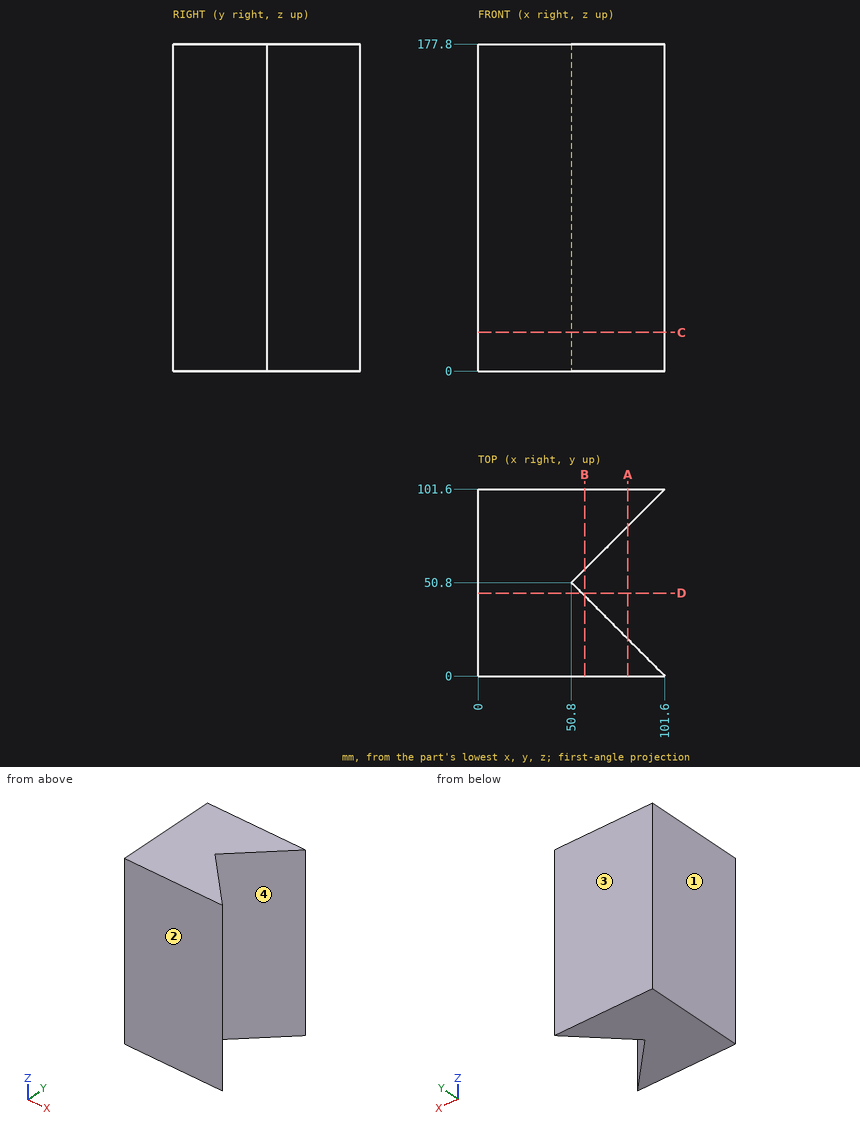
Geometry check sheet. Reference: drawing and pictorial views, mm from the part's lowest x, y, z. Round coordinates to 2 decimals unless told otherwise and drop trailing zeros. Write each loop counter-clockwise with the first axis right and the second up, starting at its lowest first coordinate (ties: lowest second). Pieces come first, ordered by that corner, then holes. Notation, with made-up numbers: (-40, -25.5) -> (-33, -25.5) arc R30 cw to (-33, 6.5) -> close; hole circle Ø10 at (-0.5, 6.5). An arc over 180 degrees is marked (long way). Put each result on its own line as item: value.
1) Cross-section at A-A, the plane x = 81.5. Enter the section's corners in (y, z), plus the area to 3 significant figures.
Recorded:
outline: (0, 0) -> (20.1, 0) -> (20.1, 177.8) -> (0, 177.8) -> close; (81.5, 0) -> (101.6, 0) -> (101.6, 177.8) -> (81.5, 177.8) -> close
area: 7,150 mm2
2) Depth check by flat-ended pin: P1, Ø12, axis at y = 40.5, z = 143.5, coming from the +X side; P2, Ø8, axis at x = 28, y = 47.5, coming from the -Z side. Enter the tip coordinate at first touch or a pass-through.
Recorded:
P1: stops at x = 67.1
P2: stops at z = 0
3) Cross-section at B-B, the plane x = 58. Enter the section's corners in (y, z), plus the area to 3 significant figures.
Recorded:
outline: (0, 0) -> (43.6, 0) -> (43.6, 177.8) -> (0, 177.8) -> close; (58, 0) -> (101.6, 0) -> (101.6, 177.8) -> (58, 177.8) -> close
area: 15,500 mm2
4) Release check for a two-part mould opening along Y. For the marked faces 1, 2, 3 and 4 record: pulls with the +Y half, pulls with the -Y half, needs draft (parallel to the pull), parting line crosses it, or undercut.
Recorded:
face 1: needs draft
face 2: pulls with the -Y half
face 3: pulls with the +Y half
face 4: undercut
5) Cross-section at C-C, the plane z = 21. Enter the section's corners in (x, y).
Recorded:
outline: (0, 0) -> (101.6, 0) -> (50.8, 50.8) -> (101.6, 101.6) -> (0, 101.6) -> close
6) Cross-section at D-D, the plane y = 45. Enter the section's corners in (x, z), plus the area to 3 significant figures.
Recorded:
outline: (0, 0) -> (56.6, 0) -> (56.6, 177.8) -> (0, 177.8) -> close
area: 10,100 mm2
7) Thickness scan on probe 1 along Y at (x, z) = (88.5, 96); probe 2 along Y at (x, z) = (92, 50); probe 3 along X at (y, z) = (20, 149). Record the ranges inside material, lowest first. Write a range as from..to.
Recorded:
probe 1: y = 0..13.1, 88.5..101.6
probe 2: y = 0..9.6, 92..101.6
probe 3: x = 0..81.6
